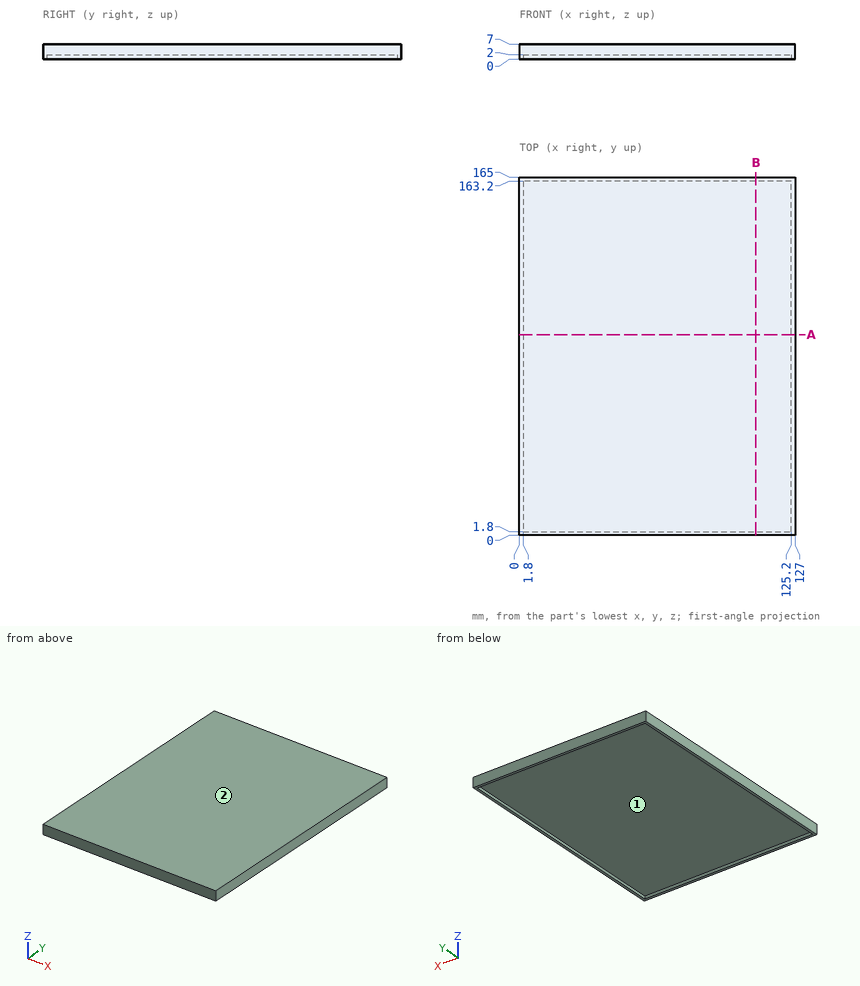
Verification items for this drawing (mm, ordinates from the low corner). Coordinates: 2 decimals unless noted, no trailing zeros. Order: outer loops, then holes, each group sorted by start corner. A loop starts at its lowest first (then second) coordinate and runs counter-clockwise, first axis right, second up. Notation, with made-up numbers: (-20, 39) -> (10, 39) arc R17 cw to (10, 70) -> close; hole circle Ø11 at (65.5, 14.5). An arc over 180 degrees is marked (long way). Answer as CSV lines item,"result". Start each with the question number.
1) Cross-section at B-B, the plane x = 109. Record the boundary of the cut face in (y, z), then the cut area to 3 significant figures.
2) Release check for a two-part mould opening along Y. For the marked faces 1 and 2 record: released by +Y, released by -Y, zero draft, split by the parting line, or undercut.
3) Cross-section at A-A, the plane y = 92.5. Record the boundary of the cut face in (x, z).
4) Material ranges on L1, parallel to X at y = 113, z = 0.75; L2, parallel to Y at x = 73.5, z = 1.25; L3, parallel to Z at x = 96, y = 10.5, recorded low to high. Write a range as [from, to].
Conclusion:
1,outline,"(0, 0) -> (1.8, 0) -> (1.8, 2) -> (163.2, 2) -> (163.2, 0) -> (165, 0) -> (165, 7) -> (0, 7) -> close"
1,area,"832 mm²"
2,face 1,"undercut"
2,face 2,"zero draft"
3,outline,"(0, 0) -> (1.8, 0) -> (1.8, 2) -> (125.2, 2) -> (125.2, 0) -> (127, 0) -> (127, 7) -> (0, 7) -> close"
4,L1,"x = [0, 1.8], [125.2, 127]"
4,L2,"y = [0, 1.8], [163.2, 165]"
4,L3,"z = [2, 7]"
